Input: part model. Units: mm. Frame: model coordinates. Round coordinates to 2 decimals unless told otherwise and drop trailing zeros. Write each loop counter-clockwise with the first axis right and the second up, starting at its lowest first coordinate (ties: lowest second). Pieces come first, ordered by that corner, then holes. Notation, with made-up numbers: (17, -38.75) -> (35, -38.75) arc R38 ccw to (35, 0.25) -> close; hole circle Ø8 at (-19.5, 69.5). An arc over 180 degrees is marked (long way). Use CSV: the item, a comma, the result in double quotes.
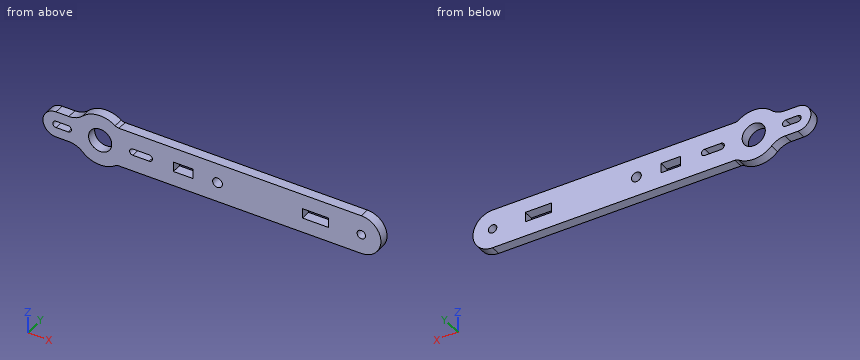
```python
from build123d import *

# Parameters (mm, degrees)
ESBO_O1_R                    = 4
ESBO_O1_R_2                  = 7.85
ESBO_O1_R_3                  = 6
RESSALTO_EXTRUS_O1_DEPTH     = 3
FURO_DE_DI_METRO_7_1_7_1_1_D = 7.1
CORTE_EXTRUS_O1_DEPTH        = 100.754611422
ESBO_O3_W                    = 8
ESBO_O3_H                    = 3
ESBO_O3_W_2                  = 6
CORTE_EXTRUS_O2_DEPTH        = 100.754611422
FURO_DE_DI_METRO_2_6_2_6_1_D = 2.6
FURO_DE_DI_METRO_3_0_3_1_D   = 3
FILETE1_R                    = 2
FILETE2_R                    = 6


with BuildPart() as part:
    # Esboço1 → Ressalto-extrusão1 (new body)
    with BuildSketch(Plane(origin=(0, 0, 0), x_dir=(1, 0, 0), z_dir=(0, 1, 0))):
        Circle(ESBO_O1_R)
        with BuildLine():
            ThreePointArc((6.745557018, -4), (5.65, 0), (6.745557018, 4))
            Line((6.745557018, 4), (0, 4))
            ThreePointArc((0, 4), (2.828427125, 2.828427125), (4, 0))
            ThreePointArc((4, 0), (2.828427125, -2.828427125), (0, -4))
            Line((0, -4), (6.745557018, -4))
        make_face()
        with Locations((13.5, 0)):
            Circle(ESBO_O1_R_2)
        with BuildLine():
            ThreePointArc((93.4, -6), (87.4, 0), (93.4, 6))
            Line((93.4, 6), (18.561867244, 6))
            ThreePointArc((18.561867244, 6), (20.618924001, 3.308084199), (21.35, 0))
            ThreePointArc((21.35, 0), (20.618924001, -3.308084199), (18.561867244, -6))
            Line((18.561867244, -6), (93.4, -6))
        make_face()
        with Locations((93.4, 0)):
            Circle(ESBO_O1_R_3)
    extrude(amount=-RESSALTO_EXTRUS_O1_DEPTH)

    # Furo de diâmetro Ø7.1 (7.1)1 (through all)
    with Locations(Plane(origin=(0, 0, 0), x_dir=(1, 0, 0), z_dir=(0, 1, 0))):
        with Locations((13.5, 0)):
            Hole(FURO_DE_DI_METRO_7_1_7_1_1_D / 2)

    # Esboço2 → Corte-extrusão1 (cut, through all)
    with BuildSketch(Plane(origin=(0, 0, 0), x_dir=(1, 0, 0), z_dir=(0, 1, 0))):
        with BuildLine():
            Line((0, 1), (3.7, 1))
            ThreePointArc((3.7, 1), (4.7, 0), (3.7, -1))
            Line((3.7, -1), (0, -1))
            ThreePointArc((0, -1), (-1, 0), (0, 1))
        make_face()
        with BuildLine():
            Line((23.5, 1), (28.5, 1))
            ThreePointArc((28.5, 1), (29.5, 0), (28.5, -1))
            Line((28.5, -1), (23.5, -1))
            ThreePointArc((23.5, -1), (22.5, 0), (23.5, 1))
        make_face()
    extrude(amount=-CORTE_EXTRUS_O1_DEPTH, mode=Mode.SUBTRACT)

    # Esboço3 → Corte-extrusão2 (cut, through all)
    with BuildSketch(Plane(origin=(0, 0, 0), x_dir=(1, 0, 0), z_dir=(0, 1, 0))):
        with Locations((79.4, 0)):
            Rectangle(ESBO_O3_W, ESBO_O3_H)
        with Locations((38.9, 0)):
            Rectangle(ESBO_O3_W_2, ESBO_O3_H)
    extrude(amount=-CORTE_EXTRUS_O2_DEPTH, mode=Mode.SUBTRACT)

    # Furo de diâmetro Ø2.6 (2.6)1 (through all)
    with Locations(Plane(origin=(0, 0, 0), x_dir=(1, 0, 0), z_dir=(0, 1, 0))):
        with Locations((93.4, 0)):
            Hole(FURO_DE_DI_METRO_2_6_2_6_1_D / 2)

    # Furo de diâmetro Ø3.0 (3)1 (through all)
    with Locations(Plane(origin=(0, 0, 0), x_dir=(1, 0, 0), z_dir=(0, 1, 0))):
        with Locations((49.4, 0)):
            Hole(FURO_DE_DI_METRO_3_0_3_1_D / 2)

    # Filete1
    filete1_edges = [part.edges().sort_by_distance(p)[0] for p in [
        (18.561867244, -1.5, -6),
        (18.561867244, -1.5, 6),
    ]]
    fillet(filete1_edges, radius=FILETE1_R)

    # Filete2
    filete2_edges = [part.edges().sort_by_distance(p)[0] for p in [
        (6.745557018, -1.5, -4),
        (6.745557018, -1.5, 4),
    ]]
    fillet(filete2_edges, radius=FILETE2_R)


solid = part.part
```
Item 1: First-contact query: pin 1 Ø1.5 at (x, y) = (2, -2) entering from +Z; pin 2 Ø1.5 at (x, y) = (59, -2) entering from -Z. Flat tips, straight axial feed; report the tip coordinate or a pass-through.
Worked answers:
pin 1,"stops at z = 4"
pin 2,"stops at z = -6"
Item 2: Line query: line 1 (Z direction, x = 93.4, y = -1.65); line 2 (Z direction, x = 49.4, y = -2.1); line 3 (Z direction, x = 89.5, y = -0.05). Output: solid intervals per line, ascending.
Worked answers:
line 1,"z = -6 to -1.3, 1.3 to 6"
line 2,"z = -6 to -1.5, 1.5 to 6"
line 3,"z = -6 to 6"
Item 3: Section query A-A on z = 0. Give the number of separate pieces and of enclosed holes in the cut face, plus the area to 3 significant figures.
Worked answers:
separate pieces,"8"
enclosed holes,"0"
area,"192 mm²"
Item 4: Section query D-D on x = 13.5. Return the cut outline in (y, z).
Worked answers:
outline,"(-3, -7.85) -> (0, -7.85) -> (0, -3.55) -> (-3, -3.55) -> close; (-3, 3.55) -> (0, 3.55) -> (0, 7.85) -> (-3, 7.85) -> close"
Item 5: Section query B-B on x = 49.4. Return the cut outline in (y, z).
Worked answers:
outline,"(-3, -6) -> (0, -6) -> (0, -1.5) -> (-3, -1.5) -> close; (-3, 1.5) -> (0, 1.5) -> (0, 6) -> (-3, 6) -> close"
